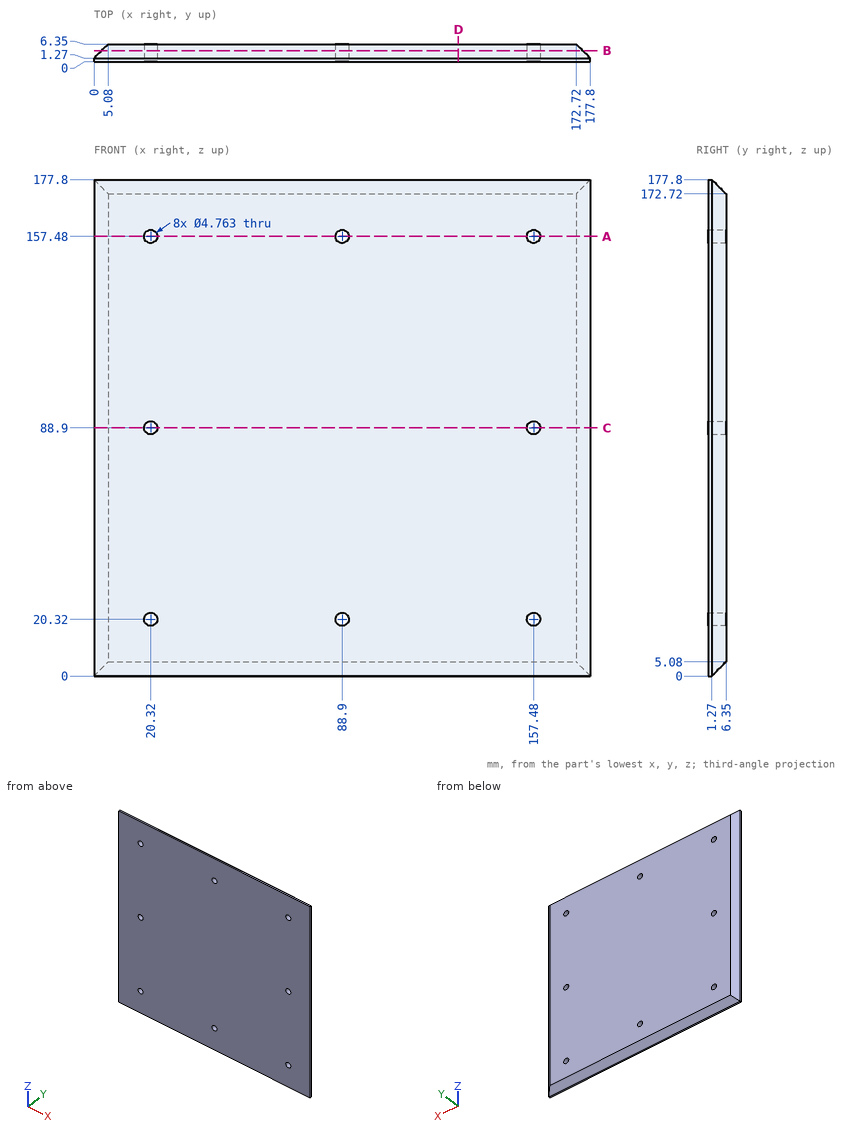
Answer from the drawing. Dimensions are ordinates in mm from the lowest x, y and z of the part. Round coordinates to 2 decimals unless told otherwise and drop trailing zeros. Loops run counter-clockwise (first coordinate to the right, second up) from the corner with the lowest first, then second, coordinate; pieces in that order, holes last. Notation, with made-up numbers: (37, 88) - (86, 88) arc R27 cw to (86, 123) - close; hole circle Ø3 at (-39.75, 59). An arc over 180 degrees is marked (long way). Return JSON: item names as keys, results as strings. Group by question number.
1. The part is cut by section C-C on z = 88.9. Determine the outline of the cut face in (x, y), then the cut area to 3 significant figures.
2. Consider probe 1 along X at (y, z) = (2.75, 20.32); probe 2 along X at (y, z) = (4, 88.9); probe 3 along X at (y, z) = (5.25, 88.9). Determine where each line is inside the solid, lowest interval first.
3. Each of these flat-tipped pins is pushed along its axis until it touches: P1, Ø2, axis at x = 143, y = 4, coming from the +Z side; P2, Ø3, axis at x = 88.9, z = 157.48, coming from the -Y side; P3, Ø2, axis at x = 119.5, y = 2.5, coming from the +Z side. Where does it stop, or does it pass through?
4. The part is cut by section A-A on z = 157.48. Determine the outline of the cut face in (x, y), then the cut area to 3 significant figures.
5. The part is cut by section B-B on y = 4. State how many separate pieces and enclosed holes the cut face has, then the cut area to 3 significant figures.
6. The part is cut by section D-D on x = 130.5. Determine the outline of the cut face in (y, z).
Resolved:
{
 "1": {"outline": "(0, 0) - (17.94, 0) - (17.94, 6.35) - (5.08, 6.35) - (0, 1.27) - close; (22.7, 0) - (155.1, 0) - (155.1, 6.35) - (22.7, 6.35) - close; (159.86, 0) - (177.8, 0) - (177.8, 1.27) - (172.72, 6.35) - (159.86, 6.35) - close", "area": "1,040 mm²"},
 "2": {"probe 1": "x = 1.48 to 17.94, 22.7 to 86.52, 91.28 to 155.1, 159.86 to 176.32", "probe 2": "x = 2.73 to 17.94, 22.7 to 155.1, 159.86 to 175.07", "probe 3": "x = 3.98 to 17.94, 22.7 to 155.1, 159.86 to 173.82"},
 "3": {"P1": "stops at z = 176.07", "P2": "passes through", "P3": "stops at z = 177.57"},
 "4": {"outline": "(0, 0) - (17.94, 0) - (17.94, 6.35) - (5.08, 6.35) - (0, 1.27) - close; (22.7, 0) - (86.52, 0) - (86.52, 6.35) - (22.7, 6.35) - close; (91.28, 0) - (155.1, 0) - (155.1, 6.35) - (91.28, 6.35) - close; (159.86, 0) - (177.8, 0) - (177.8, 1.27) - (172.72, 6.35) - (159.86, 6.35) - close", "area": "1,010 mm²"},
 "5": {"separate pieces": "1", "enclosed holes": "8", "area": "29,600 mm²"},
 "6": {"outline": "(0, 0) - (1.27, 0) - (6.35, 5.08) - (6.35, 172.72) - (1.27, 177.8) - (0, 177.8) - close"}
}
